Geometry check sheet. Reference: drawing and pictorial views, mm from the part's lowest x, y, z. A direction names the side the tool comes from. Give positions to 0.01 mm unless a question says otherwise; leave off trailing zeros. Order: outer loops, then holes, each group sorted by start corner. A loop starts at its lowest first (then second) coordinate and runs counter-clockwise, first axis right, second up. Notation, with made-up numbers: (89, 61) - (113, 61) arc R28 cw to (113, 87) - close; hole circle Ø9 at (70.5, 52). An arc over 180 degrees is marked (long way). Answer as a JSON object with one key per item and string values.
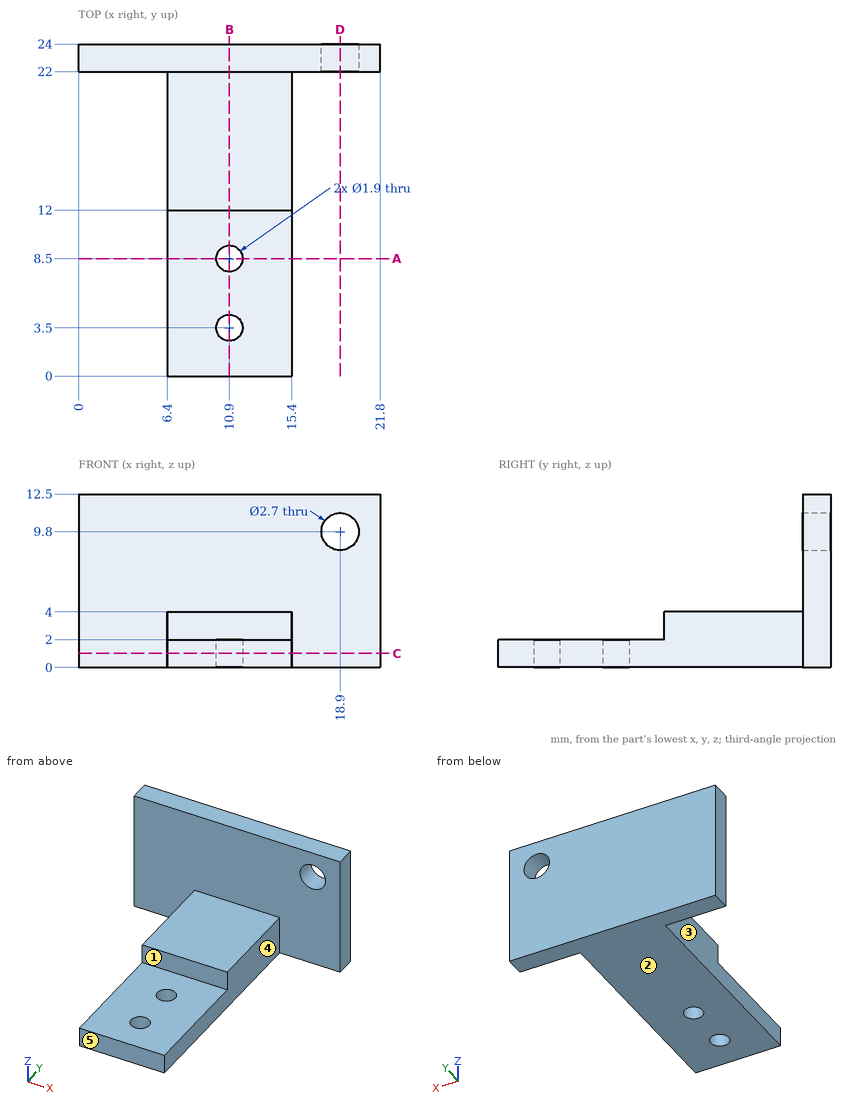
(1) Material ranges on line 1 along Y through (x, z) = (10.9, 0.6); line 2 along Z through (x, y) = (18.9, 23.1); line 3 along Y through (x, z) = (17.5, 8.25), recorded low to high. Write a range as [from, to].
Computed values:
{"line 1": "y = [0, 2.55], [4.45, 7.55], [9.45, 24]", "line 2": "z = [0, 8.45], [11.15, 12.5]", "line 3": "y = [22, 24]"}
(2) Section check D-D (x = 18.9). Record the cut outline in (y, z), then the cut area to 3 significant figures.
Computed values:
{"outline": "(22, 0) - (24, 0) - (24, 8.45) - (22, 8.45) - close; (22, 11.15) - (24, 11.15) - (24, 12.5) - (22, 12.5) - close", "area": "19.6 mm²"}
(3) Access from +Z, -Z, +X, -X, +Y, -Y to the whole of each face (thin tool, end or side, straight path). Record for the marked faces 1, 2, 3, 4 and 5.
Computed values:
{"face 1": "+Z, +X, -X, -Y", "face 2": "-Z, +X, -X, +Y, -Y", "face 3": "+Z, -Z, -X, -Y", "face 4": "+Z, -Z, +X, -Y", "face 5": "+Z, -Z, +X, -X, -Y"}
(4) Section check C-C (z = 1). Record the cut outline in (x, y), then the cut area to 3 significant figures.
Computed values:
{"outline": "(0, 22) - (6.4, 22) - (6.4, 0) - (15.4, 0) - (15.4, 22) - (21.8, 22) - (21.8, 24) - (0, 24) - close; hole circle Ø1.9 at (10.9, 3.5); hole circle Ø1.9 at (10.9, 8.5)", "area": "236 mm²"}
(5) Section check A-A (y = 8.5). Record the cut outline in (x, z), then the cut area to 3 significant figures.
Computed values:
{"outline": "(6.4, 0) - (9.95, 0) - (9.95, 2) - (6.4, 2) - close; (11.85, 0) - (15.4, 0) - (15.4, 2) - (11.85, 2) - close", "area": "14.2 mm²"}
(6) Gauge pin test, flat ends, axial feed: pin 1 Ø2.5 at (x, y) = (10.5, 15.5) entering from +Z; pin 2 Ø1.5 at (x, z) = (2.5, 1.5) entering from -Y; pin 3 Ø2.5 at (x, z) = (18.9, 9.8) entering from -Y; pin 4 Ø8 at (x, y) = (11, 12.5) entering from -Z. Record the tip position at first contact, or that the pin passes through.
Computed values:
{"pin 1": "stops at z = 4", "pin 2": "stops at y = 22", "pin 3": "passes through", "pin 4": "stops at z = 0"}
(7) Section check B-B (x = 10.9). Record the cut outline in (y, z).
Computed values:
{"outline": "(0, 0) - (2.55, 0) - (2.55, 2) - (0, 2) - close; (4.45, 0) - (7.55, 0) - (7.55, 2) - (4.45, 2) - close; (9.45, 0) - (24, 0) - (24, 12.5) - (22, 12.5) - (22, 4) - (12, 4) - (12, 2) - (9.45, 2) - close"}
